Work out the finished part from the listing and answer in its coordinate system (mm). Coordinates: 2 decimals unless noted, no trailing zeros. Loops run counter-clockwise (first coordinate to the right, second up) from the corner with the lowest first, then second, coordinate; pieces in that order, holes last. Notation, with made-up numbers: (87.5, 87) -> (93.5, 87) arc R35 cw to (93.5, 123) -> close; hole circle Ø7 at (-16.5, 14). An arc over 180 degrees is marked (long way). Answer as CSV lines item,"result".
```python
from build123d import *

# Parameters (mm, degrees)
F0_W     = 30
F0_H     = 30
F1_DEPTH = 220
F2_R     = 5
F3_R     = 14
F4_DEPTH = 40


with BuildPart() as f1:
    # F0 (on Front) → F1 (new body)
    with BuildSketch(Plane.XZ):
        Rectangle(F0_W, F0_H)
    extrude(amount=F1_DEPTH)

    # F2
    f2_edges = [f1.edges().sort_by_distance(p)[0] for p in [
        (15, -220, 0),
        (-15, -220, 0),
        (0, -220, 15),
        (0, -220, -15),
    ]]
    fillet(f2_edges, radius=F2_R)

    # F3 (on face) → F4 (cut)
    with BuildSketch(Plane.YZ.offset(15)):
        with Locations((-183.8199943304, 0)):
            Circle(F3_R)
    extrude(amount=-F4_DEPTH, mode=Mode.SUBTRACT)


solid = f1.part
```
(1) A flat-ended cylindrical pin translates along its axis: pin 1 Ø8 at (x, z) = (9.5, 6.5) entering from +Y. Find the tip coordinate at first contact, or state that the pin passes through.
Computed values:
pin 1,"y = 0"
(2) A cutting plane is placed at D-D, the plane x = -13. Write down the section's boundary in (y, z).
Computed values:
outline,"(-219, -13) arc R5 ccw to (-215, -15) -> (0, -15) -> (0, 15) -> (-215, 15) arc R5 ccw to (-219, 13) -> close; hole circle Ø28 at (-183.82, 0)"
(3) A cutting plane is placed at C-C, the plane y = -192. Write down the section's boundary in (x, z), and give its area (3 significant figures).
Computed values:
outline,"(-15, -15) -> (15, -15) -> (15, -11.36) -> (-15, -11.36) -> close; (-15, 11.36) -> (15, 11.36) -> (15, 15) -> (-15, 15) -> close"
area,"218 mm2"
(4) A cutting plane is placed at A-A, the plane x = 0.75. Write down the section's boundary in (y, z).
Computed values:
outline,"(-220, -10) arc R5 ccw to (-215, -15) -> (0, -15) -> (0, 15) -> (-215, 15) arc R5 ccw to (-220, 10) -> close; hole circle Ø28 at (-183.82, 0)"
(5) A cutting plane is placed at B-B, the plane z = 0. Write down the section's boundary in (x, y), and give its area (3 significant figures).
Computed values:
outline,"(-15, -215) arc R5 ccw to (-10, -220) -> (10, -220) arc R5 ccw to (15, -215) -> (15, -197.82) -> (-15, -197.82) -> close; (-15, -169.82) -> (15, -169.82) -> (15, 0) -> (-15, 0) -> close"
area,"5,750 mm2"
(6) Consider line 1 along Y through (x, z) = (6.5, -9.25); line 2 along Y through (x, z) = (6, -11.75); line 3 along Z through (x, y) = (-10.5, -188.5). Determine where each line is inside the solid, lowest interval first.
Computed values:
line 1,"-220 to -194.33, -173.31 to 0"
line 2,"-219.68 to -191.43, -176.21 to 0"
line 3,"-15 to -13.19, 13.19 to 15"
(7) For a pull along Y with two mould halves and no side action, classify faces 1 (the face through (0, 0, 0)), 2 (the face through (0, -218, -14)), 3 (the face through (0.21, -170.47, 4.21)), 4 (the face through (15, -106, 0)) as pulls with the +Y half, pulls with the -Y half, needs draft (parallel to the pull), parting line crosses it, or undercut.
Computed values:
face 1,"pulls with the +Y half"
face 2,"pulls with the -Y half"
face 3,"undercut"
face 4,"needs draft"
